The listing builds one solid part. Answer for the finished solid, in the listing's coordinates (mm). A direction names the side the tool comes from. Round coordinates to 2 decimals unless told otherwise and drop trailing zeros. Answer as a JSON object with one key per item and string values.
```python
from build123d import *

# Parameters (mm, degrees)
SKETCH_2_OUTSIDE_W  = 14.48
SKETCH_2_OUTSIDE_H  = 14.48
CUT_EXTRUDE_1_DEPTH = 18.8
CHAMFER_1_SIZE      = 0.7


with BuildPart() as part:
    # Эскиз1 → Повернуть1 (revolve)
    with BuildSketch(Plane.XY):
        Polygon((-12.8, 0), (-12.8, 4.04), (-10, 4.04), (-10, 2), (6, 2), (6, 0), align=None)
    revolve(axis=Axis((-21.700276243, 0, 0), (1, 0, 0)))

    # Эскиз2 outside → Вырез-Вытянуть1 (cut)
    with BuildSketch(Plane.ZY.offset(12.8)):
        Rectangle(SKETCH_2_OUTSIDE_W, SKETCH_2_OUTSIDE_H)
        Polygon((0, 4.041451884), (-3.5, 2.020725942), (-3.5, -2.020725942), (0, -4.041451884), (3.5, -2.020725942), (3.5, 2.020725942), align=None, mode=Mode.SUBTRACT)
    extrude(amount=-CUT_EXTRUDE_1_DEPTH, mode=Mode.SUBTRACT)

    # Фаска1
    chamfer_1_edges = [part.edges().sort_by_distance(p)[0] for p in [
        (6, -2, 0),
    ]]
    chamfer(chamfer_1_edges, length=CHAMFER_1_SIZE)

    # Эскиз5 → Вырез-Повернуть1 (revolve, cut)
    with BuildSketch(Plane(origin=(0, 0, 0), x_dir=(-1, 0, 0), z_dir=(0, 0.5, -0.866025404))):
        Polygon((12.8, 3.497483906), (12.8, 6.497483906), (11.067949192, 6.497483906), align=None)
    revolve(axis=Axis((0, 0, 0), (-1, 0, 0)), mode=Mode.SUBTRACT)


solid = part.part
```
Item 1: Which of the six approach directions +Z, -Z, +X, -X, +Y, -Y give full straight-line access (tool end or side, diameter ignored) to faces 1 (the face through (-11.419, -3.045, 1.726)), 2 (the face through (-2, 0, -2))?
Values follow:
{"face 1": "+Z, +X, -X, -Y", "face 2": "+X"}
Item 2: Flat-ended cylindrical pins translate along their axes: P1, Ø4, axis at x = -5.5, y = 3, coming from the +Z side; P2, Ø1.5, axis at x = -4, z = -2.5, coming from the -Y side. Find the tip coordinate at first contact, or state that the pin passes through.
Values follow:
{"P1": "z = 1.73", "P2": "y = -0.97"}
Item 3: Straight lines are drawn through the part: line 1 (X direction, y = 0.25, z = 2.75); line 2 (Z direction, x = -11, y = -3); line 3 (Z direction, x = 2, y = -1). For each, find the intervals that lie inside material, in ascending order.
Values follow:
{"line 1": "-12.8 to -10", "line 2": "-1.8 to 1.8", "line 3": "-1.73 to 1.73"}
